Job drawing, mm, ordinate dimensions from the low corner. One solid piece. Round coordinates to 2 decimals unless told otherwise and drop trailing zeros. Loops run counter-clockwise (first coordinate to the right, second up) from the corner with the lowest first, then second, coordinate; pieces in that order, holes last.
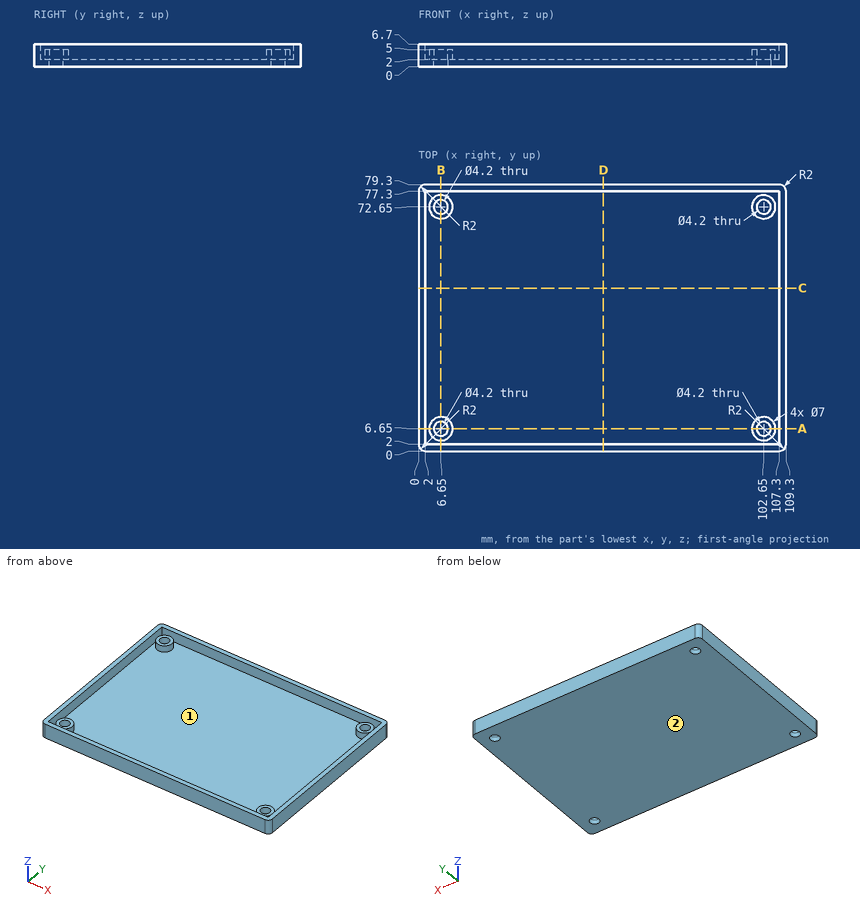
Item 1: Probe line 1 (X direction, y = 72.65, z = 0.95); line 2 (Y direction, x = 6.65, z = 0.5); line 3 (Y direction, x = 102.65, z = 2.95). List the from-to ranges inside material, lowest first.
Answers follow:
line 1: x = 0 to 4.55, 8.75 to 100.55, 104.75 to 109.3
line 2: y = 0 to 4.55, 8.75 to 70.55, 74.75 to 79.3
line 3: y = 0 to 2, 3.15 to 4.55, 8.75 to 10.15, 69.15 to 70.55, 74.75 to 76.15, 77.3 to 79.3
Item 2: Cut at D-D, the plane x = 55. Give the cut face in (y, z).
Answers follow:
outline: (0, 0) - (79.3, 0) - (79.3, 6.7) - (77.3, 6.7) - (77.3, 2) - (2, 2) - (2, 6.7) - (0, 6.7) - close
Item 3: Cut at C-C, the plane y = 48.5. Give the cut face in (x, z), plus the area to 3 significant figures.
Answers follow:
outline: (0, 0) - (109.3, 0) - (109.3, 6.7) - (107.3, 6.7) - (107.3, 2) - (2, 2) - (2, 6.7) - (0, 6.7) - close
area: 237 mm2
Item 4: Two-plate mould, pull along X, no slides. Class the marked faces 1 and 2: released by +X, released by -X, zero draft, split by the parting line, or undercut.
Answers follow:
face 1: undercut
face 2: zero draft
Item 5: Cut at A-A, the plane y = 6.65. Give the cut face in (x, z), plus the area to 3 significant figures.
Answers follow:
outline: (0, 0) - (4.55, 0) - (4.55, 5) - (3.15, 5) - (3.15, 2) - (2, 2) - (2, 6.7) - (0, 6.7) - close; (8.75, 0) - (100.55, 0) - (100.55, 5) - (99.15, 5) - (99.15, 2) - (10.15, 2) - (10.15, 5) - (8.75, 5) - close; (104.75, 0) - (109.3, 0) - (109.3, 6.7) - (107.3, 6.7) - (107.3, 2) - (106.15, 2) - (106.15, 5) - (104.75, 5) - close
area: 237 mm2
Item 6: Cut at B-B, the plane x = 6.65. Give the cut face in (y, z), plus the area to 3 significant figures.
Answers follow:
outline: (0, 0) - (4.55, 0) - (4.55, 5) - (3.15, 5) - (3.15, 2) - (2, 2) - (2, 6.7) - (0, 6.7) - close; (8.75, 0) - (70.55, 0) - (70.55, 5) - (69.15, 5) - (69.15, 2) - (10.15, 2) - (10.15, 5) - (8.75, 5) - close; (74.75, 0) - (79.3, 0) - (79.3, 6.7) - (77.3, 6.7) - (77.3, 2) - (76.15, 2) - (76.15, 5) - (74.75, 5) - close
area: 177 mm2
Item 7: Flat gauge pins, fed straight in: P1, Ø2, axis at x = 18.5, y = 14.5, coming from the +Z side; P2, Ø3.5, axis at x = 6.5, y = 5.5, coming from the +Z side. Where does each tip first touch, or does it go through?
Answers follow:
P1: stops at z = 2
P2: stops at z = 5
